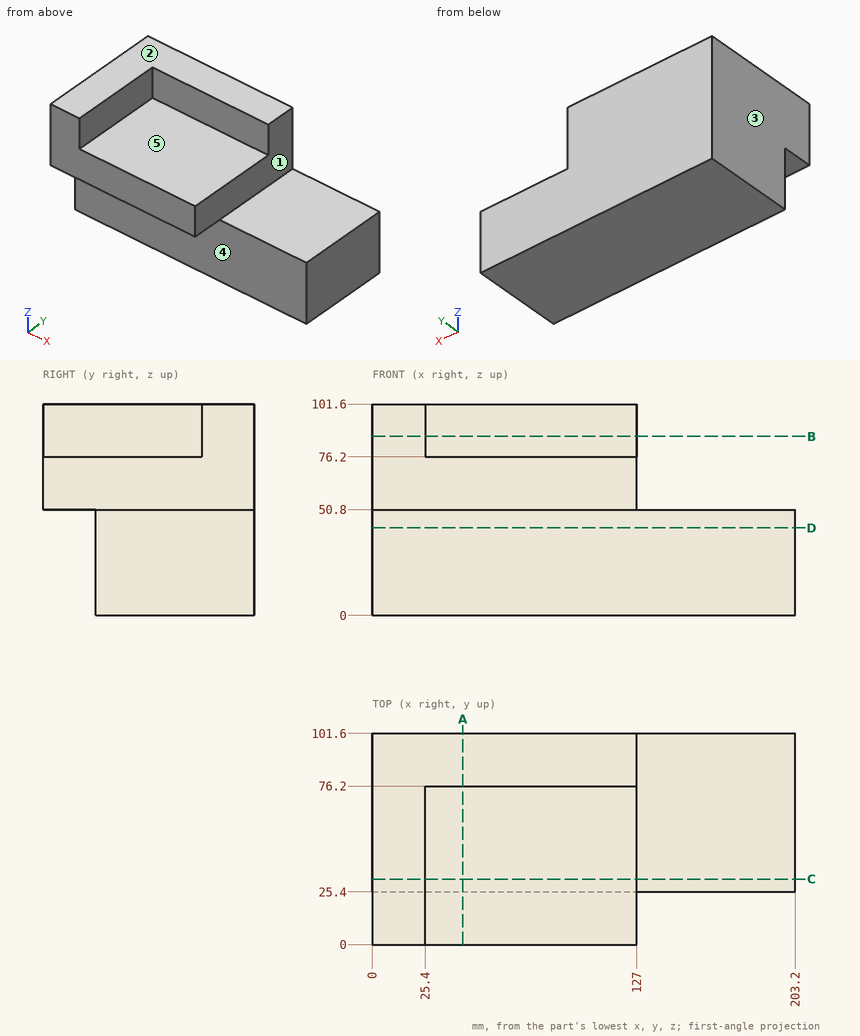
Verification items for this drawing (mm, ordinates from the low corner). A direction names the side the tool comes from. Give positions to 0.01 mm unless a question says otherwise; leave off trailing zeros. Order: outer loops, then holes, each group sorted by start corner. A loop starts at its lowest first (then second) coordinate and runs counter-clockwise, first axis right, second up.
1) Cross-section at D-D (z = 42). Record the boundary of the cut face in (x, y).
Results are:
outline: (0, 25.4) - (203.2, 25.4) - (203.2, 101.6) - (0, 101.6) - close
2) Gauge pin test, flat ends, axial feed: pin 1 (10 mm diameter, centred on x = 66.5, y = 64.5, fed in from +Z); pin 2 (20.5 mm diameter, centred on x = 40, y = 7.5, fed in from -Z); pin 3 (20.5 mm diameter, centred on y = 47.5, z = 94, fed in from +X). Record the tip position at first contact, or that the pin passes through.
Results are:
pin 1: stops at z = 76.2
pin 2: stops at z = 50.8
pin 3: stops at x = 25.4
3) Cross-section at B-B (z = 86). Record the boundary of the cut face in (x, y).
Results are:
outline: (0, 0) - (25.4, 0) - (25.4, 76.2) - (127, 76.2) - (127, 101.6) - (0, 101.6) - close
4) Cross-section at A-A (x = 43.5). Record the boundary of the cut face in (y, z).
Results are:
outline: (0, 50.8) - (25.4, 50.8) - (25.4, 0) - (101.6, 0) - (101.6, 101.6) - (76.2, 101.6) - (76.2, 76.2) - (0, 76.2) - close
5) Material ranges on probe 1 along X at (y, z) = (62.5, 56); probe 2 along Y at (x, z) = (17, 25.5); probe 3 along Z at (x, y) = (40, 70.5), recorded low to high.
Results are:
probe 1: x = 0 to 127
probe 2: y = 25.4 to 101.6
probe 3: z = 0 to 76.2
6) Cross-section at C-C (y = 31.5). Record the boundary of the cut face in (x, z).
Results are:
outline: (0, 0) - (203.2, 0) - (203.2, 50.8) - (127, 50.8) - (127, 76.2) - (25.4, 76.2) - (25.4, 101.6) - (0, 101.6) - close
7) Tool access check on the marked faces 1, 2, 3, 4 and 5. Record the directions out of +Z, -Z, +X, -X, +Y, -Y that give a thin tool (end or side, any length) a straight path to the whole face; none if there is none.
Results are:
face 1: +Z, +X, +Y, -Y
face 2: +Z, +X, -X, +Y, -Y
face 3: +Z, -Z, -X, +Y, -Y
face 4: -Z, +X, -X, -Y
face 5: +Z, +X, -Y
